Autodesk Inventor part; units mm, degrees
ref_plane "YZ Plane" through (0, 0, 0) normal (1, 0, 0) x (0, 1, 0)
ref_plane "XZ Plane" through (0, 0, 0) normal (0, 1, 0) x (-1, 0, 0)
ref_plane "XY Plane" through (0, 0, 0) normal (0, 0, 1) x (1, 0, 0)
sketch "Sketch1" plane through (0, 0, 0) normal (1, 0, 0) x (0, 1, 0)
  line L0 (-21.5, -17.5) -> (21.5, -17.5)
  line L1 (21.5, -17.5) -> (21.5, 1.5)
  line L2 (21.5, 17.5) -> (-21.5, 17.5)
  line L3 (-21.5, 17.5) -> (-21.5, -17.5)
  line L4 (-21.5, -17.5) -> (21.5, 17.5) construction
  line L5 (21.5, -17.5) -> (-21.5, 17.5) construction
  line L6 (18.0188, 17.5) -> (28.5, 17.5)
  line L7 (28.5, 17.5) -> (28.5, 1.5)
  line L8 (28.5, 1.5) -> (21.5, 1.5)
  point P0 (0, 0)
  dimension "d0" = 43
  dimension "d1" = 35
  dimension "d2" = 50
  dimension "d3" = 16
extrude "Extrusion1" add sketch "Sketch1" along normal blind 75
sketch "Sketch2" plane through (0, 28.5, 17.5) normal (0, 1, 0) x (1, 0, 0)
  line L0 (0, 0) -> (75, 0)
  line L1 (65.4712, 0) -> (65.4712, 10)
  line L2 (65.4712, 10) -> (55, 10)
  line L3 (55, 10) -> (55, 11)
  line L4 (55, 11) -> (20, 11)
  line L5 (20, 11) -> (20, 10)
  line L6 (20, 10) -> (10.4712, 10)
  line L7 (10.4712, 10) -> (10.4712, 0)
  line L8 (0, 35) -> (75, 35)
  line L9 (37.5, 35) -> (37.5, 5.3668)
  point P0 (0, 17.5)
  dimension "d6" = 55
  dimension "d7" = 35
  dimension "d8" = 17.5
  dimension "d9" = 11
  dimension "d10" = 10
extrude "Extrusion2" cut sketch "Sketch2" against normal blind 75
sketch "Sketch3" plane through (0, 21.5, 1.5) normal (0, 1, 0) x (1, 0, 0)
  circle A0 centre (10, 10) radius 5.5
  circle A1 centre (65, 10) radius 5.5
  line L0 (0, 19) -> (75, 19)
  line L1 (75, 19) -> (75, 0)
  line L2 (0, -16) -> (10.4712, -16)
  line L3 (65.4712, -16) -> (75, -16)
  point P0 (0, 1.5)
  dimension "d13" = 11
  dimension "d14" = 11
  dimension "d15" = 55
  dimension "d19" = 26
  dimension "d20" = 26
extrude "Extrusion3" cut sketch "Sketch3" against normal blind 7
sketch "Sketch4" plane through (65, 14.5, -8.5) normal (0, 1, 0) x (1, 0, 0)
  circle A0 centre (0, 0) radius 5.5
  circle A1 centre (0, 0) radius 3.2
  circle A2 centre (-55, 0) radius 5.5
  circle A3 centre (-55, 0) radius 3.2
  point P0 (-65, -8.5)
  dimension "d23" = 6.4
  dimension "d24" = 6.4
extrude "Extrusion4" cut sketch "Sketch4" against normal blind 40 contours A1 | A3
sketch "Sketch7" plane through (0, -21.5, 17.5) normal (0, 0, 1) x (1, 0, 0)
  line L0 (0, 0) -> (10.4712, 0)
  line L1 (0, 50) -> (10.4712, 50)
  point P0 (0, 21.5)
  point P1 (4.3276, 7)
  point P2 (4.6222, 43)
  point P3 (5.2356, 0)
  dimension "d31" = 7
  dimension "d32" = 36
  dimension "d33" = 7
hole "Hole1" at (4.3276, -14.5, 17.5) at (4.6222, 21.5, 17.5) direction (0, 0, -1) diameter 4.134 depth 14.2 tip angle 118
pattern_linear "Rectangular Pattern1" count 2 spacing 65 along (1, 0, 0) of "Hole1"
sketch "Sketch9" plane through (0, -21.5, -17.5) normal (0, -1, 0) x (1, 0, 0)
  circle A0 centre (37.5, 11) radius 6
  line L0 (0, 35) -> (0, 0)
  line L1 (0, 35) -> (10.4712, 35)
  point P0 (0, 17.5)
  dimension "d53" = 37.5
  dimension "d54" = 24
  dimension "d55" = 12
extrude "Extrusion6" cut sketch "Sketch9" against normal blind 20
sketch "Sketch10" plane through (0, -21.5, -17.5) normal (0, 0, -1) x (-1, 0, 0)
  line L0 (0, 0) -> (0, 43)
  line L1 (0, 0) -> (-75, 0)
  line L2 (-75, 0) -> (-75, 43)
  point P0 (0, 21.5)
  point P1 (-34, 7)
  dimension "d59" = 7
  dimension "d60" = 41
hole "Hole3" at (34, -14.5, -17.5) direction (0, 0, 1) diameter 2.459 depth 8.8 tip angle 118
properties part number "Lose Backe"
Verification items for the finished model (mm, model axes). A direction names the side the tool comes from. Give positions to 0.01 mm unless a question says otherwise; leave off trailing zeros. Order: outer loops, then holes, each group sorted by start corner. A loop starts at its lowest first (then second) coordinate and runs counter-clockwise, first axis right, second up. Notation, with made-up numbers: M 34,68.5 L 78,68.5 A21 cw 78,74.5 Z; hole C 19,29 d7. An arc over 180 degrees is marked long. Use one line per item in the form item = value. Start each with the question number.
Q1. Section check A-A (z = 12.5). Enter the section's corners in (x, y), then the cut area to 3 significant figures.
Q2. Section check B-B (x = 8.5). Enter the section's corners in (y, z), then the cut area to 3 significant figures.
Q3. Scan lines: line 1 along X through (y, z) = (4, -8.5); line 2 along X through (y, z) = (18.5, -8.5); line 3 along X through (y, z) = (-14.5, 8). Record each from-to range of solid material in increasing order. Write a range as [from, to].
Q4. Go/stop test with flat-tipped pins: pin 1 Ø9 at (x, z) = (65, -8.5) entering from +Y; pin 2 Ø6 at (x, z) = (12.5, -7.5) entering from +Y; pin 3 Ø2 at (x, y) = (34, -14.5) entering from -Z. Record where each tip stops, or that it passes through.
Q5. Mould release check, pull along X, two halves, no side actions. Record for faces 6 (the flat face through (70, 4, 17.5)), 7 (the flat face through (0, 3, 0)), 8 (the flat face through (75, 3, 0)), 9 (the conical face through (4.6, 21.9, 2.3)): +X half, -X half, draft (parallel to the pull), parting line (faces both ways), or undercut.
Q6. Access from +Z, -Z, +X, -X, +Y, -Y to the whole of each face (thin tool, end or side, straight path). Record for faces 1 (the flat face through (37, 21.5, -8)), 2 (the flat face through (37, -1.5, -6)), 3 (the flat face through (12.4, 14.5, -6.1)), 4 (the flat face through (60, 4, 7.5)), 5 (the cylindrical face through (71.46, 20.55, 10.3)).
Q7. Section check C-C (x = 37.5). Enter the section's corners in (y, z).
Q8. Section check D-D (z = -8.5). Enter the section's corners in (x, y), then the cut area to 3 significant figures.
Evaluation:
q1.outline = M 0,-21.5 L 10.47,-21.5 L 10.47,28.5 L 0,28.5 Z; M 65.47,-21.5 L 75,-21.5 L 75,28.5 L 65.47,28.5 Z; hole C 4.33,-14.5 d4.13; hole C 4.62,21.5 d4.13; hole C 69.33,-14.5 d4.13; hole C 69.62,21.5 d4.13
q1.area = 946 mm2
q2.outline = M -21.5,-17.5 L 21.5,-17.5 L 21.5,-13.79 L 14.5,-13.79 L 14.5,-11.33 L -21.5,-11.33 Z; M -21.5,-5.67 L 14.5,-5.67 L 14.5,-3.21 L 21.5,-3.21 L 21.5,1.5 L 28.5,1.5 L 28.5,17.5 L -21.5,17.5 Z
q2.area = 1,340 mm2
q3.line_1 = [0, 6.8], [13.2, 61.8], [68.2, 75]
q3.line_2 = [0, 4.5], [15.5, 59.5], [70.5, 75]
q3.line_3 = [0, 2.26], [6.39, 10.47], [65.47, 67.26], [71.39, 75]
q4.pin_1 = 14.5
q4.pin_2 = 21.5
q4.pin_3 = -2.53
q5.face_6 = draft
q5.face_7 = -X half
q5.face_8 = +X half
q5.face_9 = undercut
q6.face_1 = -Z, +X, -X, +Y
q6.face_2 = -Y
q6.face_3 = +Y
q6.face_4 = +Z, +Y, -Y
q6.face_5 = +Z
q7.outline = M -21.5,-17.5 L 21.5,-17.5 L 21.5,1.5 L 28.5,1.5 L 28.5,6.5 L -21.5,6.5 L -21.5,-0.5 L -1.5,-0.5 L -1.5,-12.5 L -21.5,-12.5 Z
q8.outline = M 0,-21.5 L 6.8,-21.5 L 6.8,14.5 L 4.5,14.5 L 4.5,21.5 L 0,21.5 Z; M 13.2,-21.5 L 31.84,-21.5 L 31.84,-1.5 L 43.16,-1.5 L 43.16,-21.5 L 61.8,-21.5 L 61.8,14.5 L 59.5,14.5 L 59.5,21.5 L 15.5,21.5 L 15.5,14.5 L 13.2,14.5 Z; M 68.2,-21.5 L 75,-21.5 L 75,21.5 L 70.5,21.5 L 70.5,14.5 L 68.2,14.5 Z
q8.area = 2,380 mm2
